Geometry: final body of the model. Coordinates: model frame, mm. A direction names the side the tool comes from. Coordinates: 2 decimals unless noted, no trailing zeros. Write each loop counter-clockwise with the first axis right and the second up, starting at its lowest first coordinate (ties: lowest second). Pieces come first, ordered by that corner, then holes. Notation, with made-up numbers: (84, 78) - (102, 78) arc R8 cw to (102, 89) - close; hole circle Ø4 at (40.5, -20). An arc over 180 degrees is marked (long way). Answer as a JSON object with one key per item and string values. Group by question number.
Item 1: First-contact query: pin 1 Ø1.3 at (y, z) = (-1, 36.5) entering from -X. Flat tip, straight axial feed; report the tip coordinate or a pass-through.
Item 2: Section A-A on x = 0. Return loops of the section in (y, z), and give its area (3 significant figures).
Item 3: Mould query, pull axis X, two halves, no side actions, for faces 5 (the flat face through (6.5, -3, 47)), 6 (the flat face through (8.5, -5, 47)), 7 (the flat face through (5, 8.5, 47)). Classes: pulls with the +X half, pulls with the -X half, needs draft (parallel to the pull), parting line crosses it, or undercut.
Item 4: Set-up query: faces 1 (the flat face through (-5, 8.5, 47)), 2 (the flat face through (-1.5, 8, 47)), 3 (the flat face through (-1.5, -7, 47)), 4 (the flat face through (4.805, 3.39, 46.835)). Return all of +Z, -Z, +X, -X, +Y, -Y with unobstructed straight access to the full face (end or side cutting, diameter ignored); none if empty.
Item 5: Line query: line 1 along X through (y, z) = (3.25, 30); line 2 along Y through (x, z) = (7, 20); line 3 along Y through (x, z) = (-1.75, 19.5). Output: solid intervals per line, ascending. Write a range as from..to.
```python
from build123d import *

# Parameters (mm, degrees)
SKETCH1_R           = 1.5
BOSS_EXTRUDE1_DEPTH = 95


with BuildPart() as part:
    # Sketch1 → Boss-Extrude1 (new body)
    with BuildSketch(Plane.XY):
        with BuildLine():
            Line((-2.085786438, 3.5), (2.085786438, 3.5))
            Line((2.085786438, 3.5), (4.659009742, 6.073223305))
            ThreePointArc((4.659009742, 6.073223305), (4.71320293, 6.345670858), (4.482233047, 6.5))
            Line((4.482233047, 6.5), (1.75, 6.5))
            ThreePointArc((1.75, 6.5), (1.573223305, 6.573223305), (1.5, 6.75))
            Line((1.5, 6.75), (1.5, 8.25))
            ThreePointArc((1.5, 8.25), (1.573223305, 8.426776695), (1.75, 8.5))
            Line((1.75, 8.5), (8.25, 8.5))
            ThreePointArc((8.25, 8.5), (8.426776695, 8.426776695), (8.5, 8.25))
            Line((8.5, 8.25), (8.5, 1.75))
            ThreePointArc((8.5, 1.75), (8.426776695, 1.573223305), (8.25, 1.5))
            Line((8.25, 1.5), (6.75, 1.5))
            ThreePointArc((6.75, 1.5), (6.573223305, 1.573223305), (6.5, 1.75))
            Line((6.5, 1.75), (6.5, 4.482233047))
            ThreePointArc((6.5, 4.482233047), (6.345670858, 4.71320293), (6.073223305, 4.659009742))
            Line((6.073223305, 4.659009742), (3.5, 2.085786438))
            Line((3.5, 2.085786438), (3.5, -2.085786438))
            Line((3.5, -2.085786438), (6.073223305, -4.659009742))
            ThreePointArc((6.073223305, -4.659009742), (6.345670858, -4.71320293), (6.5, -4.482233047))
            Line((6.5, -4.482233047), (6.5, -1.75))
            ThreePointArc((6.5, -1.75), (6.573223305, -1.573223305), (6.75, -1.5))
            Line((6.75, -1.5), (8.25, -1.5))
            ThreePointArc((8.25, -1.5), (8.426776695, -1.573223305), (8.5, -1.75))
            Line((8.5, -1.75), (8.5, -8.25))
            ThreePointArc((8.5, -8.25), (8.426776695, -8.426776695), (8.25, -8.5))
            Line((8.25, -8.5), (1.75, -8.5))
            ThreePointArc((1.75, -8.5), (1.573223305, -8.426776695), (1.5, -8.25))
            Line((1.5, -8.25), (1.5, -6.75))
            ThreePointArc((1.5, -6.75), (1.573223305, -6.573223305), (1.75, -6.5))
            Line((1.75, -6.5), (4.482233047, -6.5))
            ThreePointArc((4.482233047, -6.5), (4.71320293, -6.345670858), (4.659009742, -6.073223305))
            Line((4.659009742, -6.073223305), (2.085786438, -3.5))
            Line((2.085786438, -3.5), (-2.085786438, -3.5))
            Line((-2.085786438, -3.5), (-4.659009742, -6.073223305))
            ThreePointArc((-4.659009742, -6.073223305), (-4.71320293, -6.345670858), (-4.482233047, -6.5))
            Line((-4.482233047, -6.5), (-1.75, -6.5))
            ThreePointArc((-1.75, -6.5), (-1.573223305, -6.573223305), (-1.5, -6.75))
            Line((-1.5, -6.75), (-1.5, -8.25))
            ThreePointArc((-1.5, -8.25), (-1.573223305, -8.426776695), (-1.75, -8.5))
            Line((-1.75, -8.5), (-8.25, -8.5))
            ThreePointArc((-8.25, -8.5), (-8.426776695, -8.426776695), (-8.5, -8.25))
            Line((-8.5, -8.25), (-8.5, -1.75))
            ThreePointArc((-8.5, -1.75), (-8.426776695, -1.573223305), (-8.25, -1.5))
            Line((-8.25, -1.5), (-6.75, -1.5))
            ThreePointArc((-6.75, -1.5), (-6.573223305, -1.573223305), (-6.5, -1.75))
            Line((-6.5, -1.75), (-6.5, -4.482233047))
            ThreePointArc((-6.5, -4.482233047), (-6.345670858, -4.71320293), (-6.073223305, -4.659009742))
            Line((-6.073223305, -4.659009742), (-3.5, -2.085786438))
            Line((-3.5, -2.085786438), (-3.5, 2.085786438))
            Line((-3.5, 2.085786438), (-6.073223305, 4.659009742))
            ThreePointArc((-6.073223305, 4.659009742), (-6.345670858, 4.71320293), (-6.5, 4.482233047))
            Line((-6.5, 4.482233047), (-6.5, 1.75))
            ThreePointArc((-6.5, 1.75), (-6.573223305, 1.573223305), (-6.75, 1.5))
            Line((-6.75, 1.5), (-8.25, 1.5))
            ThreePointArc((-8.25, 1.5), (-8.426776695, 1.573223305), (-8.5, 1.75))
            Line((-8.5, 1.75), (-8.5, 8.25))
            ThreePointArc((-8.5, 8.25), (-8.426776695, 8.426776695), (-8.25, 8.5))
            Line((-8.25, 8.5), (-1.75, 8.5))
            ThreePointArc((-1.75, 8.5), (-1.573223305, 8.426776695), (-1.5, 8.25))
            Line((-1.5, 8.25), (-1.5, 6.75))
            ThreePointArc((-1.5, 6.75), (-1.573223305, 6.573223305), (-1.75, 6.5))
            Line((-1.75, 6.5), (-4.482233047, 6.5))
            ThreePointArc((-4.482233047, 6.5), (-4.71320293, 6.345670858), (-4.659009742, 6.073223305))
            Line((-4.659009742, 6.073223305), (-2.085786438, 3.5))
        make_face()
        Circle(SKETCH1_R, mode=Mode.SUBTRACT)
    extrude(amount=BOSS_EXTRUDE1_DEPTH)


solid = part.part
```
Checks:
{
 "1": {"pin 1": "x = -8.48"},
 "2": {"outline": "(-3.5, 0) - (-1.5, 0) - (-1.5, 95) - (-3.5, 95) - close; (1.5, 0) - (3.5, 0) - (3.5, 95) - (1.5, 95) - close", "area": "380 mm^2"},
 "3": {"face 5": "undercut", "face 6": "pulls with the +X half", "face 7": "needs draft"},
 "4": {"face 1": "+Z, -Z, +X, -X, +Y", "face 2": "+Z, -Z, +Y", "face 3": "+Z, -Z, -Y", "face 4": "+Z, -Z"},
 "5": {"line 1": "-8.5..-6.5, -4.66..4.66, 6.5..8.5", "line 2": "-8.5..-1.5, 1.5..8.5", "line 3": "-8.5..-6.5, -3.5..3.5, 6.5..8.5"}
}
